For this review, take the finished solid that the model builds, in its own axes (mm). A direction names the side the tool comes from. Coordinates: 2 decimals unless noted, no trailing zeros. Return JSON: item names as keys, results as strings.
```python
from build123d import *

# Parameters (mm, degrees)
FILLET2_R       = 0.5
SKETCH2_W       = 3.2
SKETCH2_H       = 0.4
SLOT_DEPTH      = 0.35
THDSCHPAT_COUNT = 22
THDSCHPAT_PITCH = 0.347619048


with BuildPart() as part:
    # BodySke → Base-Revolve (revolve)
    with BuildSketch(Plane.XY, mode=Mode.PRIVATE) as base_revolve_sk:
        Polygon((1, 0.8), (1, 1.6), (0, 1.512511336), (0, 0), (9, 0), (9, 0.8), align=None)
    revolve(base_revolve_sk.sketch.rotate(Axis((-25.4, 0, 0), (1, 0, 0)), 90), axis=Axis((-25.4, 0, 0), (1, 0, 0)))

    # Fillet2
    fillet2_edges = [part.edges().sort_by_distance(p)[0] for p in [
        (0, 0, -1.512511336),
    ]]
    fillet(fillet2_edges, radius=FILLET2_R)

    # Sketch2 → Slot (cut)
    with BuildSketch(Plane(origin=(0, 0, 0), x_dir=(0, 0, -1), z_dir=(1, 0, 0))):
        Rectangle(SKETCH2_W, SKETCH2_H)
    extrude(amount=SLOT_DEPTH, mode=Mode.SUBTRACT)

    # ThdSchSke → ThreadSchematic (revolve, cut)
    with BuildSketch(Plane.XY):
        Polygon((1.7, -0.601), (1.5606587, -0.8), (1.5606587, -1), (1.8393413, -1), (1.8393413, -0.8), align=None)
    threadschematic = revolve(axis=Axis((-3.175, 0, 0), (1, 0, 0)), mode=Mode.SUBTRACT)

    # ThdSchPat: ThreadSchematic ×22
    with Locations(*[(i * THDSCHPAT_PITCH, 0, 0) for i in range(1, THDSCHPAT_COUNT)]):
        add(threadschematic, mode=Mode.SUBTRACT)


solid = part.part
```
1. For faces 1 (the face through (0, -0.5, 0)), 2 (the face through (1, -1, 0)), list the 3-axis set-ups (+Z, -Z, +X, -X, +Y, -Y) from which the entire face can be reached by the end or side of a thin tool; tool diameter is ignored.
Checks:
{"face 1": "+Z, -Z, -X, +Y, -Y", "face 2": "+X"}
2. Wall thickness on L1, parallel to X at y = -0.9, z = -0.05; L2, parallel to Z at x = 1.25, y = 0.1; L3, parallel to X at y = 1.2, z = 0.85: over which ranges is each line inside the solid? List them lowest first. Write a range as from..to.
Checks:
{"L1": "0..1", "L2": "-0.79..0.79", "L3": "0.22..1"}
3. Clearance check with flat-ended pins moving along their axes: pin 1 Ø1.5 at (x, z) = (2, 1) entering from +Y; pin 2 Ø1.5 at (x, y) = (1.5, 1) entering from -Z. State where each tip first meets the part, or that it passes through.
Checks:
{"pin 1": "y = 0.76", "pin 2": "z = -1.54"}
